Could you check a few things on this model? Use its own coordinates, in mm. A direction names the side the tool comes from. Give positions to 0.01 mm unless a question says otherwise; leave off trailing zeros. Order: outer loops, then holes, each group sorted by start corner. A loop starts at its lowest first (then second) coordinate and runs counter-clockwise, first axis right, second up. Notation, with made-up numbers: M 28,-10 L 77,-10 A19 cw 77,3 Z; hole C -3,1.5 d1. An arc over 180 degrees is marked long. Use a Markdown table: item, result. Add a question column.
Item 1: Suppose I cut it at C-C on z = 12. Write out the boundary of the cut face in (x, y), plus the area to 3 significant figures.
Item 2: Suppose I cut it at A-A on x = 26.67. Write out the boundary of the cut face in (y, z), plus the area to 3 significant figures.
Item 3: Suppose I cut it at B-B on x = 39. Write out the boundary of the cut face in (y, z).
Item 4: For faces 1 (the face through (-23.935, 63.678, 18.313)), 2 (the face through (45.593, 3, 35)), 3 (the face through (-17.701, 39, -15)), which set-ups out of +Z, -Z, +X, -X, +Y, -Y let a thin tool reach every point of the face, with its end or its side?
Item 5: Suppose I cut it at D-D on y = 24. Write out the boundary of the cut face in (x, z).
Item 6: If I drill on L1, parallel to X at y = 2, z = -37; L2, parallel to X at y = 3, z = -37.38; L3, parallel to Z at x = 7, y = 45.5, over which ranges is the centre line in solid material (lowest first)? Write a range as from..to.
Item 7: If we mould it in two halves opening along Z, with no side actions, what happens to faces 4 (the face through (14, 76.2, -21)), 5 (the face through (-25, 50.8, -18)), 6 (the face through (6, 3, -45))? For each: released by +Z, released by -Z, zero draft, split by the parting line, or undercut.
Item 8: I'm going to push flat-ended pins straight in: pin 1 Ø2.5 at (y, z) = (1.5, -32.5) entering from +X; pin 2 Ø11 at (x, y) = (-23.5, 38.5) entering from +Z; pin 3 Ø1.8 at (x, z) = (-25.321, -17.822) entering from +Y; pin 4 Ø7 at (x, z) = (26.67, 37.38) entering from +Y (3 decimals). Where does each tip first touch, or does it pass through?
from build123d import *

# Parameters (mm, degrees)
SKETCH1_W                    = 91.186
SKETCH1_H                    = 90
SKETCH1_R                    = 3.96875
MOUNTING_PLATE_EXTRUDE_DEPTH = 5.08
SKETCH3_W                    = 102.41
SKETCH3_H                    = 50.8
MAIN_EXTRUDE_DEPTH           = 71.12
SKETCH4_W                    = 23.876
SKETCH4_H                    = 50.8
BOSS_EXTRUDE3_DEPTH          = 5.08
SKETCH5_R                    = 1.5
CUT_EXTRUDE1_DEPTH           = 25.4
SKETCH7_W                    = 12.652
SKETCH7_H                    = 90
CUT_EXTRUDE3_DEPTH           = 5.08
CUT_EXTRUDE4_DEPTH           = 5.08


with BuildPart() as part:
    # Sketch1 → Mounting plate extrude (new body)
    with BuildSketch(Plane(origin=(0, 0, 0), x_dir=(1, 0, 0), z_dir=(0, 1, 0))):
        Rectangle(SKETCH1_W, SKETCH1_H)
        with Locations((26.67, -37.38)):
            Circle(SKETCH1_R, mode=Mode.SUBTRACT)
        with Locations((-11.684, -37.38)):
            Circle(SKETCH1_R, mode=Mode.SUBTRACT)
        with Locations((-11.684, 37.38)):
            Circle(SKETCH1_R, mode=Mode.SUBTRACT)
        with Locations((26.67, 37.38)):
            Circle(SKETCH1_R, mode=Mode.SUBTRACT)
    extrude(amount=MOUNTING_PLATE_EXTRUDE_DEPTH)

    # Sketch3 → Main extrude (add)
    with BuildSketch(Plane(origin=(0, 5.08, 0), x_dir=(1, 0, 0), z_dir=(0, 1, 0))):
        with Locations((18.264, 0.042)):
            Rectangle(SKETCH3_W, SKETCH3_H)
        Polygon((-17.701, 9.567), (-17.701, 20.362), (63.579, 20.362), (63.579, 9.567), (63.579, -9.483), (63.579, -20.278), (-17.701, -20.278), (-17.701, -9.483), (-27.861, -9.483), (-27.861, 9.567), align=None, mode=Mode.SUBTRACT)
    extrude(amount=MAIN_EXTRUDE_DEPTH)

    # Sketch4 → Boss-Extrude3 (add)
    with BuildSketch(Plane.XZ.offset(-5.08)):
        with Locations((57.531, -0.042)):
            Rectangle(SKETCH4_W, SKETCH4_H)
    extrude(amount=BOSS_EXTRUDE3_DEPTH)

    # Sketch5 → Cut-Extrude1 (cut)
    with BuildSketch(Plane(origin=(0, 76.2, 0), x_dir=(1, 0, 0), z_dir=(0, 1, 0))):
        with Locations((-25.321, 17.822)):
            Circle(SKETCH5_R)
        with Locations((-25.321, -17.738)):
            Circle(SKETCH5_R)
    extrude(amount=-CUT_EXTRUDE1_DEPTH, mode=Mode.SUBTRACT)

    # Sketch7 → Cut-Extrude3 (cut)
    with BuildSketch(Plane(origin=(0, 5.08, 0), x_dir=(1, 0, 0), z_dir=(0, 1, 0))):
        with Locations((-39.267, 0)):
            Rectangle(SKETCH7_W, SKETCH7_H)
    extrude(amount=-CUT_EXTRUDE3_DEPTH, mode=Mode.SUBTRACT)

    # Sketch8 → Cut-Extrude4 (cut)
    with BuildSketch(Plane(origin=(0, 5.08, 0), x_dir=(1, 0, 0), z_dir=(0, 1, 0))):
        Polygon((-17.701, 20.362), (-17.701, 9.567), (-27.861, 9.567), (-27.861, -9.483), (-17.701, -9.483), (-17.701, -20.278), (63.579, -20.278), (63.579, 20.362), align=None)
    extrude(amount=-CUT_EXTRUDE4_DEPTH, mode=Mode.SUBTRACT)


solid = part.part
Findings below:
| question | item | result |
|---|---|---|
| 1 | outline | M -32.94,0 L -17.7,0 L -17.7,76.2 L -32.94,76.2 Z; M 63.58,0 L 69.47,0 L 69.47,76.2 L 63.58,76.2 Z |
| 1 | area | 1,610 mm^2 |
| 2 | outline | M 0,-45 L 5.08,-45 L 5.08,-41.35 L 0,-41.35 Z; M 0,-33.41 L 5.08,-33.41 L 5.08,-25.44 L 76.2,-25.44 L 76.2,-20.36 L 0,-20.36 Z; M 0,20.28 L 76.2,20.28 L 76.2,25.36 L 5.08,25.36 L 5.08,33.41 L 0,33.41 Z; M 0,41.35 L 5.08,41.35 L 5.08,45 L 0,45 Z |
| 2 | area | 893 mm^2 |
| 3 | outline | M 0,-45 L 5.08,-45 L 5.08,-25.44 L 76.2,-25.44 L 76.2,-20.36 L 0,-20.36 Z; M 0,20.28 L 76.2,20.28 L 76.2,25.36 L 5.08,25.36 L 5.08,45 L 0,45 Z |
| 4 | face 1 | +Y |
| 4 | face 2 | +Z, +X, +Y, -Y |
| 4 | face 3 | +Y, -Y |
| 5 | outline | M -32.94,-25.44 L 69.47,-25.44 L 69.47,25.36 L -32.94,25.36 Z; hole M -27.86,-9.57 L -17.7,-9.57 L -17.7,-20.36 L 63.58,-20.36 L 63.58,20.28 L -17.7,20.28 L -17.7,9.48 L -27.86,9.48 Z |
| 6 | L1 | x = -32.94..-15.63, -7.73..22.72, 30.62..45.59 |
| 6 | L2 | x = -32.94..-15.65, -7.72..22.7, 30.64..45.59 |
| 6 | L3 | z = -25.44..-20.36, 20.28..25.36 |
| 7 | face 4 | zero draft |
| 7 | face 5 | undercut |
| 7 | face 6 | released by -Z |
| 8 | pin 1 | stops at x = 45.59 |
| 8 | pin 2 | stops at z = 25.36 |
| 8 | pin 3 | stops at y = 50.8 |
| 8 | pin 4 | passes through |
